Design review of the part built by this model. Coordinates are the model's own, in mm. Round coordinates to 2 decimals unless told otherwise and drop trailing zeros. Order: outer loops, then holes, each group sorted by start corner. A loop starts at its lowest first (then second) coordinate and runs counter-clockwise, first axis right, second up. Notation, with made-up numbers: M 79,56 L 83,56 A11 ccw 83,72 Z; hole C 61,-34.75 d4. An arc over 180 degrees is marked long. Write each question's results on one line, items separated by ' | '. Start each with the question number.
Item 1: Take a section at D-D, the plane x = 9. Write out the cut boundary in (y, z).
Item 2: Take a section at A-A, the plane y = -6.5. Write out the cut boundary in (x, z), plus the area to 3 significant figures.
Item 3: Clearance check with flat-ended pins moving along their axes: pin 1 (0.5 mm diameter, centred on x = -34.5, z = 1, fed in from -Y); pin 2 (1.2 mm diameter, centred on x = 33, y = -9.33, fed in from -Z); pin 3 (1.5 mm diameter, centred on y = -16.5, z = 2, fed in from -X); pin 4 (1.5 mm diameter, centred on y = -20.5, z = 2, fed in from +X). State where each tip first meets the part, or that it passes through.
Item 4: Wall thickness on line 1 (X direction, y = -65, z = 1.4); line 2 (Y direction, x = 23, z = 1.5); line 3 (Y direction, x = 10, z = 0.35): over which ranges is each line inside the solid? List them lowest first. Write a range as [from, to].
Item 5: Take a section at C-C, the plane z = 0.6. Count the separate pieces of the cut face and the enclosed holes in it, plus the area to 3 significant figures.
Item 6: Take a section at B-B, the plane x = -16. Write out the cut boundary in (y, z).
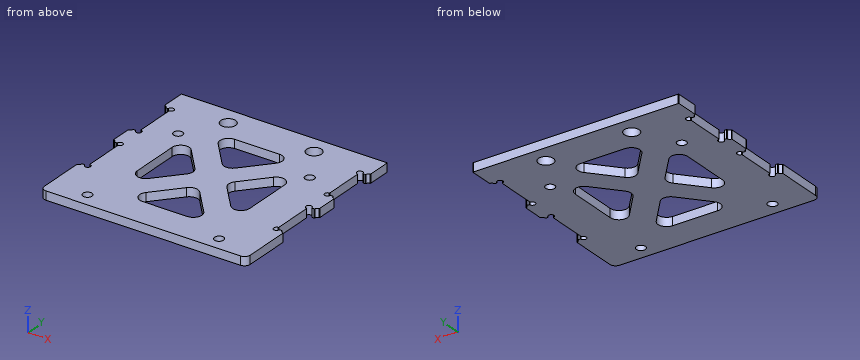
```python
from build123d import *
from OCP.BRepFilletAPI import BRepFilletAPI_MakeFillet

# Parameters (mm, degrees)
SKETCH_1_R          = 2.6
SKETCH_1_W          = 72
SKETCH_1_H          = 10
EXTRUDE_1_DEPTH     = 3
FILLET_1_R1         = 0.2
FILLET_1_R2         = 2
SKETCH_2_R          = 1.6
CUT_EXTRUDE_1_DEPTH = 10
SKETCH_8_R          = 1.6
CUT_EXTRUDE_5_DEPTH = 3
SKETCH_10_R         = 1.6
CUT_EXTRUDE_6_DEPTH = 10
SKETCH_11_W         = 39.340466826
SKETCH_11_H         = 45.8017909
CUT_EXTRUDE_7_DEPTH = 10
EXTRUDE_1_2_DEPTH   = 3
FILLET_2_R          = 3


with BuildPart() as part:
    # Sketch 1 → Extrude 1 (new body)
    # profile 1 of 2: a face of its own
    with BuildSketch(Plane.XY):
        with BuildLine():
            Line((36, 0), (-36, 0))
            Line((-36, 0), (-36, -8.333333333))
            ThreePointArc((-36, -8.333333333), (-35.292893219, -8.626226552), (-35, -9.333333333))
            Line((-35, -9.333333333), (-34, -9.333333333))
            ThreePointArc((-34, -9.333333333), (-33, -8.333333333), (-32, -9.333333333))
            ThreePointArc((-32, -9.333333333), (-32.292893219, -10.040440115), (-33, -10.333333333))
            Line((-33, -10.333333333), (-33, -24.333333333))
            ThreePointArc((-33, -24.333333333), (-32.292893219, -24.626226552), (-32, -25.333333333))
            ThreePointArc((-32, -25.333333333), (-33, -26.333333333), (-34, -25.333333333))
            Line((-34, -25.333333333), (-35, -25.333333333))
            ThreePointArc((-35, -25.333333333), (-35.292893219, -26.040440115), (-36, -26.333333333))
            Line((-36, -26.333333333), (-36, -33.666666667))
            ThreePointArc((-36, -33.666666667), (-35.292893219, -33.959559885), (-35, -34.666666667))
            Line((-35, -34.666666667), (-34, -34.666666667))
            ThreePointArc((-34, -34.666666667), (-33, -33.666666667), (-32, -34.666666667))
            ThreePointArc((-32, -34.666666667), (-32.292893219, -35.373773448), (-33, -35.666666667))
            Line((-33, -35.666666667), (-33, -49.666666667))
            ThreePointArc((-33, -49.666666667), (-32.292893219, -49.959559885), (-32, -50.666666667))
            ThreePointArc((-32, -50.666666667), (-33, -51.666666667), (-34, -50.666666667))
            Line((-34, -50.666666667), (-35, -50.666666667))
            ThreePointArc((-35, -50.666666667), (-35.292893219, -51.373773448), (-36, -51.666666667))
            Line((-36, -51.666666667), (-36, -60))
            Line((-36, -60), (36, -60))
            Line((36, -60), (36, -51.666666667))
            ThreePointArc((36, -51.666666667), (35.292893219, -51.373773448), (35, -50.666666667))
            Line((35, -50.666666667), (34, -50.666666667))
            ThreePointArc((34, -50.666666667), (32.292893219, -51.373773448), (33, -49.666666667))
            Line((33, -49.666666667), (33, -35.666666667))
            ThreePointArc((33, -35.666666667), (32.292893219, -33.959559885), (34, -34.666666667))
            Line((34, -34.666666667), (35, -34.666666667))
            ThreePointArc((35, -34.666666667), (35.292893219, -33.959559885), (36, -33.666666667))
            Line((36, -33.666666667), (36, -26.333333333))
            ThreePointArc((36, -26.333333333), (35.292893219, -26.040440115), (35, -25.333333333))
            Line((35, -25.333333333), (34, -25.333333333))
            ThreePointArc((34, -25.333333333), (32.292893219, -26.040440115), (33, -24.333333333))
            Line((33, -24.333333333), (33, -10.333333333))
            ThreePointArc((33, -10.333333333), (32.292893219, -8.626226552), (34, -9.333333333))
            Line((34, -9.333333333), (35, -9.333333333))
            ThreePointArc((35, -9.333333333), (35.292893219, -8.626226552), (36, -8.333333333))
            Line((36, -8.333333333), (36, 0))
        make_face()
        with Locations((-15, -6.5)):
            Circle(SKETCH_1_R, mode=Mode.SUBTRACT)
        with Locations((15, -6.5)):
            Circle(SKETCH_1_R, mode=Mode.SUBTRACT)
    # profile 2 of 2: a face of its own
    with BuildSketch(Plane.XY):
        with Locations((0, -65)):
            Rectangle(SKETCH_1_W, SKETCH_1_H)
    extrude(amount=EXTRUDE_1_DEPTH)

    # Fillet 1: one fillet with a radius per group of edges: ONE call of the kernel's fillet builder (fillet() takes one radius for all edges)
    fillet_1_edges_1 = [part.edges().sort_by_distance(p)[0] for p in [
        (-35, -9.333333333, 1.5),
        (-34, -9.333333333, 1.5),
        (33, -10.333333333, 1.5),
        (34, -9.333333333, 1.5),
        (35, -9.333333333, 1.5),
        (36, -8.333333333, 1.5),
        (36, 0, 1.5),
        (-36, 0, 1.5),
        (-36, -8.333333333, 1.5),
        (-33, -10.333333333, 1.5),
        (-33, -24.333333333, 1.5),
        (-34, -25.333333333, 1.5),
        (-35, -25.333333333, 1.5),
        (-36, -26.333333333, 1.5),
        (-36, -33.666666667, 1.5),
        (-35, -34.666666667, 1.5),
        (-34, -34.666666667, 1.5),
        (-33, -35.666666667, 1.5),
        (-33, -49.666666667, 1.5),
        (-34, -50.666666667, 1.5),
        (-35, -50.666666667, 1.5),
        (-36, -51.666666667, 1.5),
        (36, -51.666666667, 1.5),
        (35, -50.666666667, 1.5),
        (34, -50.666666667, 1.5),
        (33, -49.666666667, 1.5),
        (33, -35.666666667, 1.5),
        (34, -34.666666667, 1.5),
        (35, -34.666666667, 1.5),
        (36, -33.666666667, 1.5),
        (36, -26.333333333, 1.5),
        (35, -25.333333333, 1.5),
        (34, -25.333333333, 1.5),
        (33, -24.333333333, 1.5),
    ]]
    fillet_1_edges_2 = [part.edges().sort_by_distance(p)[0] for p in [
        (-36, -70, 1.5),
        (36, -70, 1.5),
    ]]
    fillet_1 = BRepFilletAPI_MakeFillet(part.part.solid().wrapped)
    for e in fillet_1_edges_1:
        fillet_1.Add(FILLET_1_R1, e.wrapped)
    for e in fillet_1_edges_2:
        fillet_1.Add(FILLET_1_R2, e.wrapped)
    add(Compound.cast(fillet_1.Shape()), mode=Mode.REPLACE)

    # Sketch 2 → Cut-Extrude 1 (cut)
    with BuildSketch(Plane.XY.offset(3)):
        with Locations((-23, -20)):
            Circle(SKETCH_2_R)
        with Locations((23, -20)):
            Circle(SKETCH_2_R)
    extrude(amount=-CUT_EXTRUDE_1_DEPTH, mode=Mode.SUBTRACT)

    # Sketch 8 → Cut-Extrude 5 (cut)
    with BuildSketch(Plane.XY.offset(3)):
        with Locations((23, -65)):
            Circle(SKETCH_8_R)
        with Locations(Location((-23, -65, 0), (0, 0, 180))):
            Circle(SKETCH_8_R)
    extrude(amount=-CUT_EXTRUDE_5_DEPTH, mode=Mode.SUBTRACT)

    # Sketch 10 → Cut-Extrude 6 (cut)
    with BuildSketch(Plane.XY.offset(3)):
        with Locations((-12, -30)):
            Circle(SKETCH_10_R)
        with Locations((-12, -40)):
            Circle(SKETCH_10_R)
        with Locations((12, -40)):
            Circle(SKETCH_10_R)
        with Locations((12, -30)):
            Circle(SKETCH_10_R)
    extrude(amount=-CUT_EXTRUDE_6_DEPTH, mode=Mode.SUBTRACT)

    # Sketch 11 → Cut-Extrude 7 (cut)
    with BuildSketch(Plane.XY.offset(3)):
        with Locations((0, -36.393264277)):
            Rectangle(SKETCH_11_W, SKETCH_11_H)
    extrude(amount=-CUT_EXTRUDE_7_DEPTH, mode=Mode.SUBTRACT)

    # Sketch 12 → Extrude 1 2 (add)
    with BuildSketch(Plane.XY.offset(3)):
        Polygon((17.282301657, -10.133497371), (-23.728051839, -57.879439072), (-17.659356964, -63.092014492), (23.350996533, -15.346072791), align=None)
        Polygon((-23.419012344, -15.266885984), (17.312700126, -62.688422331), (23.381395001, -57.475846911), (-17.350317469, -10.054310564), align=None)
    extrude(amount=-EXTRUDE_1_2_DEPTH)

    # Fillet 2
    fillet_2_edges = [part.edges().sort_by_distance(p)[0] for p in [
        (-14.397270996, -13.492368827, 1.5),
        (14.397270996, -13.492368827, 1.5),
        (-19.670233413, -19.631368731, 1.5),
        (-19.670233413, -53.155159823, 1.5),
        (14.397270996, -59.294159727, 1.5),
        (-14.397270996, -59.294159727, 1.5),
        (19.670233413, -53.155159823, 1.5),
        (19.670233413, -19.631368731, 1.5),
        (5.272962417, -36.393264277, 1.5),
        (0, -42.532264181, 1.5),
        (-5.272962417, -36.393264277, 1.5),
        (0, -30.254264374, 1.5),
    ]]
    fillet(fillet_2_edges, radius=FILLET_2_R)


solid = part.part
```
Results list:
1) outline: M -70,0 L -59.07,0 L -59.07,3 L -70,3 Z; M -53.01,0 L -40.73,0 L -40.73,3 L -53.01,3 Z; M -32.05,0 L -19.78,0 L -19.78,3 L -32.05,3 Z; M -13.72,0 L 0,0 L 0,3 L -13.72,3 Z
2) outline: M -36,0 L -17.6,0 L -17.6,3 L -36,3 Z; M -12.4,0 L 12.4,0 L 12.4,3 L -12.4,3 Z; M 17.6,0 L 36,0 L 36,3 L 17.6,3 Z | area: 185 mm²
3) pin 1: y = -69.98 | pin 2: through | pin 3: x = -33 | pin 4: x = 33
4) line 1: [-36, -24.6], [-21.4, 21.4], [24.6, 36] | line 2: [-70, -66.6], [-63.4, -21.6], [-18.4, 0] | line 3: [-70, -58.4], [-54.17, -41.9], [-30.89, -18.61], [-14.38, 0]
5) separate pieces: 1 | enclosed holes: 10 | area: 3,880 mm²
6) outline: M -70,0 L -47.98,0 L -47.98,3 L -70,3 Z; M -24.8,0 L -8.9,0 L -8.9,3 L -24.8,3 Z; M -4.1,0 L 0,0 L 0,3 L -4.1,3 Z
